Here's how the part is built. I have some questions about the finished solid (model axes, mm). Round coordinates to 2 decimals unless told otherwise and drop trailing zeros. Order: outer loops, then holes, each group sorted by start corner. A loop starts at its lowest first (then second) coordinate and runs counter-clockwise, first axis right, second up. Notation, with made-up numbers: (31, 13.5) - (60, 13.5) arc R29 cw to (60, 51.5) - close; hole circle Ø10 at (88, -15). An arc over 180 degrees is marked (long way). One line per item, written item: value.
from build123d import *

# Parameters (mm, degrees)
F1_DEPTH = 25.4
F2_R     = 2.413
F3_DEPTH = 12.7
F4_R     = 2.413
F5_DEPTH = 12.7


with BuildPart() as f1:
    # F0 (on Front) → F1 (new body)
    with BuildSketch(Plane.XZ):
        Polygon((-35.131108, 65.991136), (-73.231108, 0), (2.968892, 0), align=None)
    extrude(amount=F1_DEPTH)

    # F2 (on face) → F3 (cut)
    with BuildSketch(Plane.XZ.offset(25.4)):
        with Locations((-63.874334, 4.29648)):
            Circle(F2_R)
        with Locations((-48.597958, 4.29648)):
            Circle(F2_R)
        with Locations((-35.131108, 4.29648)):
            Circle(F2_R)
        with Locations((-19.763807, 4.29648)):
            Circle(F2_R)
        with Locations((-4.487435, 4.29648)):
            Circle(F2_R)
    extrude(amount=-F3_DEPTH, mode=Mode.SUBTRACT)

    # F4 (on face) → F5 (cut)
    with BuildSketch(Plane.XZ.offset(25.4)):
        with Locations((-56.427099, 18.427124)):
            Circle(F4_R)
        with Locations((-40.768821, 18.427124)):
            Circle(F4_R)
        with Locations((-27.592948, 18.427124)):
            Circle(F4_R)
        with Locations((-15.180895, 18.427124)):
            Circle(F4_R)
        with Locations((-23.391945, 32.175861)):
            Circle(F4_R)
        with Locations((-35.131108, 32.175861)):
            Circle(F4_R)
        with Locations((-49.170826, 32.175861)):
            Circle(F4_R)
        with Locations((-41.15073, 43.633141)):
            Circle(F4_R)
        with Locations((-29.120585, 43.633141)):
            Circle(F4_R)
        with Locations((-35.131108, 53.944688)):
            Circle(F4_R)
    extrude(amount=-F5_DEPTH, mode=Mode.SUBTRACT)


solid = f1.part
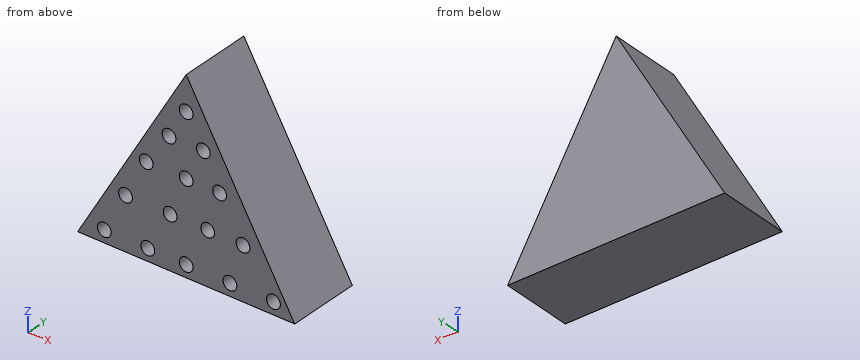
Q1. If we section it at C-C, the plane y = -10: Please give me the cut outline in (x, z).
Results list:
outline: (-73.23, 0) - (2.97, 0) - (-35.13, 65.99) - close
Q2. If I drill on line 1 along X through (y, z) = (-17.5, 45); line 2 along X through (y, z) = (-18.5, 6.5); line 3 along Z through (x, y) = (-64, -19.75), over which ranges is the centre line in solid material (lowest first)?
Results list:
line 1: -47.25 to -43.14, -39.16 to -31.11, -27.13 to -23.01
line 2: -69.48 to -64.86, -62.89 to -49.58, -47.61 to -36.11, -34.15 to -20.75, -18.78 to -5.47, -3.5 to -0.78
line 3: 0 to 1.89, 6.71 to 15.99
Q3. If we section it at A-A, the plane x = -28.5: Please give me the cut outline in (y, z).
Results list:
outline: (-25.4, 0) - (0, 0) - (0, 54.51) - (-25.4, 54.51) - (-25.4, 45.96) - (-12.7, 45.96) - (-12.7, 41.3) - (-25.4, 41.3) - (-25.4, 20.66) - (-12.7, 20.66) - (-12.7, 16.19) - (-25.4, 16.19) - close
Q4. Will these pins go through, and if not, where does the flat tip stop? pin 1 (4 mm diameter, centred on x = -19.76, z = 4.3, fed in from -Y); pin 2 (4 mm diameter, centred on y = -12, z = 32.5, fed in from +X); pin 3 (1.5 mm diameter, centred on x = -48, y = -8, fed in from +Z).
Results list:
pin 1: y = -12.7
pin 2: x = -14.64
pin 3: z = 45
Q5. If we section it at D-D, the plane x = -19: Please give me the cut outline in (y, z).
Results list:
outline: (-25.4, 0) - (0, 0) - (0, 38.05) - (-25.4, 38.05) - (-25.4, 6.59) - (-12.7, 6.59) - (-12.7, 2.01) - (-25.4, 2.01) - close
Q6. If we section it at B-B, the plane z = 20: Please give me the cut outline in (x, y), then the cut area to 3 significant figures.
Results list:
outline: (-61.68, -25.4) - (-58.26, -25.4) - (-58.26, -12.7) - (-54.6, -12.7) - (-54.6, -25.4) - (-42.6, -25.4) - (-42.6, -12.7) - (-38.94, -12.7) - (-38.94, -25.4) - (-29.42, -25.4) - (-29.42, -12.7) - (-25.76, -12.7) - (-25.76, -25.4) - (-17.01, -25.4) - (-17.01, -12.7) - (-13.35, -12.7) - (-13.35, -25.4) - (-8.58, -25.4) - (-8.58, 0) - (-61.68, 0) - close
area: 1,160 mm²
